Design review of the part built by this model. Coordinates are the model's own, in mm. Coordinates: 2 decimals unless noted, no trailing zeros. Write each loop counter-clockwise with the first axis right and the second up, starting at its lowest first coordinate (ties: lowest second). Pieces come first, ordered by that corner, then holes. Notation, with made-up numbers: (29.25, 16) - (68.25, 16) arc R20 cw to (68.25, 20) - close; hole circle Ø11 at (-35.5, -5.75). An arc over 180 degrees is marked (long way). One line per item, written item: value.
from build123d import *

# Parameters (mm, degrees)
F0_W     = 120
F0_H     = 100
F0_R     = 2
F0_R_2   = 5
F1_DEPTH = 10


with BuildPart() as f1:
    # F0 (on Front) → F1 (new body)
    with BuildSketch(Plane.XZ):
        Rectangle(F0_W, F0_H)
        with Locations((-55, -30)):
            Circle(F0_R, mode=Mode.SUBTRACT)
        with Locations((-30, -45)):
            Circle(F0_R, mode=Mode.SUBTRACT)
        with Locations((40, -45)):
            Circle(F0_R, mode=Mode.SUBTRACT)
        with Locations((-55, 30)):
            Circle(F0_R, mode=Mode.SUBTRACT)
        Circle(F0_R_2, mode=Mode.SUBTRACT)
    extrude(amount=F1_DEPTH)


solid = f1.part
1. Consider section C-C, the plane z = -45. Write out the cut boundary in (x, y).
Answer block:
outline: (-60, -10) - (-32, -10) - (-32, 0) - (-60, 0) - close; (-28, -10) - (38, -10) - (38, 0) - (-28, 0) - close; (42, -10) - (60, -10) - (60, 0) - (42, 0) - close
2. Consider section D-D, the plane x = -55. Write out the cut boundary in (y, z).
Answer block:
outline: (-10, -50) - (0, -50) - (0, -32) - (-10, -32) - close; (-10, -28) - (0, -28) - (0, 28) - (-10, 28) - close; (-10, 32) - (0, 32) - (0, 50) - (-10, 50) - close
3. Mouldability with a two-part tool opening along X and no side actions: class faces 1 (the face through (-60, -5, -1)), 2 (the face through (60, -5, -1)), 3 (the face through (-55, -5, -32)) as released by +X, released by -X, zero draft, split by the parting line, or undercut.
Answer block:
face 1: released by -X
face 2: released by +X
face 3: undercut
4. Consider section A-A, the plane z = 0. Write out the cut boundary in (x, y).
Answer block:
outline: (-60, -10) - (-5, -10) - (-5, 0) - (-60, 0) - close; (5, -10) - (60, -10) - (60, 0) - (5, 0) - close
5. Wall thickness on line 1 along Z through (x, y) = (40, -4.75); line 2 along Z through (x, y) = (-55, -2.5); line 3 along Z through (x, y) = (0, -6.5): over which ranges is each line inside the solid? List them lowest first.
Answer block:
line 1: z = -50 to -47, -43 to 50
line 2: z = -50 to -32, -28 to 28, 32 to 50
line 3: z = -50 to -5, 5 to 50
6. Consider section B-B, the plane x = -30. Write out the cut boundary in (y, z), then the cut area to 3 significant figures.
Answer block:
outline: (-10, -50) - (0, -50) - (0, -47) - (-10, -47) - close; (-10, -43) - (0, -43) - (0, 50) - (-10, 50) - close
area: 960 mm^2
